```python
from build123d import *

# Parameters (mm, degrees)
ESBO_O1_W               = 506.849315068
ESBO_O1_H               = 300
FLANGE_BASE1_DEPTH      = 2
DOBRA_START             = -150
DOBRA_ESBO_ADA1_DEPTH   = 300
DOBRA_ESBO_ADA1_2_DEPTH = 300
ESBO_O7_W               = 25
ESBO_O7_H               = 30
ESBO_O7_H_2             = 40
CORTE_EXTRUS_O1_DEPTH   = 409.841691807


# Read off the part's stored shape, not the designer's step: Dobra esboçada1
# Sheet-metal steps are written as plain solids
with BuildPart() as part:
    # Esboço1 → Flange-base1 (new body)
    with BuildSketch(Plane(origin=(0, 0, 0), x_dir=(1, 0, 0), z_dir=(0, 1, 0))):
        Rectangle(ESBO_O1_W, ESBO_O1_H)
    extrude(amount=-FLANGE_BASE1_DEPTH)

    # Dobra esboçada1 outline → Dobra esboçada1 (cut)
    with BuildSketch(Plane.XY.offset(DOBRA_START)):
        with BuildLine():
            Line((253.424657534, 0), (205.876233143, 0))
            Line((205.876233143, 0), (204.677764726, -1.198468417))
            ThreePointArc((204.677764726, -1.198468417), (203.78994779, -1.791688729), (202.742696309, -2))
            Line((202.742696309, -2), (253.424657534, -2))
            Line((253.424657534, -2), (253.424657534, 0))
        make_face()
    extrude(amount=DOBRA_ESBO_ADA1_DEPTH, mode=Mode.SUBTRACT)

    # Dobra esbo_ada1 2 outline → Dobra esbo_ada1 2 (add)
    with BuildSketch(Plane.XY.offset(DOBRA_START)):
        with BuildLine():
            Line((238.136670816, 35.088864797), (203.263551164, 0.215745145))
            ThreePointArc((203.263551164, 0.215745145), (203.024580925, 0.056070336), (202.742696309, 0))
            Line((202.742696309, 0), (205.876233143, 0))
            Line((205.876233143, 0), (239.550884379, 33.674651235))
            Line((239.550884379, 33.674651235), (238.136670816, 35.088864797))
        make_face()
    extrude(amount=DOBRA_ESBO_ADA1_2_DEPTH)

    # Esboço7 → Corte-extrusão1 (cut, through all)
    with BuildSketch(Plane(origin=(101.52390301, -101.52390301, 0), x_dir=(0.7071067811865464, 0.7071067811865488, 0), z_dir=(-0.7071067811865488, 0.7071067811865464, 0))):
        with Locations((180.699629026, 135)):
            Rectangle(ESBO_O7_W, ESBO_O7_H)
        with Locations((180.699629026, 0)):
            Rectangle(ESBO_O7_W, ESBO_O7_H_2)
        with Locations((180.699629026, -135)):
            Rectangle(ESBO_O7_W, ESBO_O7_H)
    extrude(amount=-CORTE_EXTRUS_O1_DEPTH, mode=Mode.SUBTRACT)


solid = part.part
```
Can you work these out from the model? Positions are in its coordinate system, mm. A direction names the side the tool comes from. Round coordinates to 2 decimals unless told otherwise and drop trailing zeros. Loops run counter-clockwise (first coordinate to the right, second up) from the corner with the lowest first, then second, coordinate; pieces in that order, holes last. Notation, with made-up numbers: (22.5, -22) -> (49.5, -22) arc R10 ccw to (49.5, -15) -> close; hole circle Ø1 at (-37.5, -30.75). An arc over 180 degrees is marked (long way). One line per item, written item: value. Start each with the question number.
1. If we mould it in two halves opening along Z, with no side actions, what happens to faces 1 (the flat face through (230, 25, -20)), 2 (the flat face through (230, 25, 20)), 3 (the flat face through (-16.9, -0.2, -150)), 4 (the flat face through (-29, -2, -2))? For each: pulls with the +Z half, pulls with the -Z half, needs draft (parallel to the pull), parting line crosses it, or undercut.
2. For faces 5 (the flat face through (-16.9, -0.2, 150)), 6 (the flat face through (-29, 0, -2)), which set-ups out of +Z, -Z, +X, -X, +Y, -Y let a thin tool reach every point of the face, with its end or its side?
3. If we section it at B-B, the plane y = 26.5: Write out the boundary of the cut face in (x, z).
4. If we section it at D-D, the plane z = -104: Write out the boundary of the cut face in (x, y).
5. If we section it at C-C, the plane x = -43: Write out the boundary of the cut face in (y, z).
6. If we section it at A-A, the plane z = -5: Write out the boundary of the cut face in (x, y), then the cut area to 3 significant figures.
7. If I drill on probe 1 along Y at (x, z) = (49, 40.5); probe 2 along X at (y, z) = (13.5, -45.5); probe 3 along X at (y, z) = (27.5, 115.5), over which ranges is the centre line in solid material (lowest first)?
8. For pin 1 (10 mm diameter, centred on y = 11.5, z = -28.5, fed in from -X); pin 2 (21 mm diameter, centred on x = 232, y = 29, fed in from +Z); pin 3 (1 mm diameter, centred on y = 18, z = -40.5, fed in from -X), each with a flat end and sliding along its axis, tell me the tip position at first contact or that it passes through.
Calculated:
1. face 1: undercut
1. face 2: undercut
1. face 3: pulls with the -Z half
1. face 4: needs draft
2. face 5: +Z, +X, -X, +Y, -Y
2. face 6: +Z, -Z, -X, +Y
3. outline: (229.55, -120) -> (232.38, -120) -> (232.38, -20) -> (229.55, -20) -> close; (229.55, 20) -> (232.38, 20) -> (232.38, 120) -> (229.55, 120) -> close
4. outline: (-253.42, -2) -> (202.74, -2) arc R2.74 ccw to (204.68, -1.2) -> (239.55, 33.67) -> (238.14, 35.09) -> (203.26, 0.22) arc R0.74 cw to (202.74, 0) -> (-253.42, 0) -> close
5. outline: (-2, -150) -> (0, -150) -> (0, 150) -> (-2, 150) -> close
6. outline: (-253.42, -2) -> (202.74, -2) arc R2.74 ccw to (204.68, -1.2) -> (221.87, 16) -> (220.46, 17.41) -> (203.26, 0.22) arc R0.74 cw to (202.74, 0) -> (-253.42, 0) -> close
6. area: 964 mm²
7. probe 1: y = -2 to 0
7. probe 2: x = 216.55 to 219.38
7. probe 3: x = 230.55 to 233.38
8. pin 1: stops at x = 209.55
8. pin 2: stops at z = 120
8. pin 3: stops at x = 220.55
